from build123d import *

# Parameters (mm, degrees)
SKETCH1_W                        = 35
SKETCH1_H                        = 38
BASE_FLANGE1_DEPTH               = 2
TAP_DRILL_FOR_M3X0_5_TAP1_D      = 2.5
FILLET1_R                        = 3
TAP_DRILL_FOR_M10X1_5_TAP1_D     = 8.5
TAP_DRILL_FOR_M10X1_5_TAP1_DEPTH = 5
TAP_DRILL_FOR_M10X1_5_TAP1_TIP   = 2.553657631


# Sheet-metal steps are written as plain solids
with BuildPart() as part:
    # Sketch1 → Base-Flange1 (new body)
    with BuildSketch(Plane(origin=(0, 0, 0), x_dir=(1, 0, 0), z_dir=(0, 1, 0))):
        Rectangle(SKETCH1_W, SKETCH1_H)
    extrude(amount=-BASE_FLANGE1_DEPTH)

    # Tap Drill for M3x0.5 Tap1 (through all)
    with Locations(Plane(origin=(0, 0, 0), x_dir=(1, 0, 0), z_dir=(0, 1, 0))):
        with Locations((-9.5, -13), (-9.5, 13)):
            Hole(TAP_DRILL_FOR_M3X0_5_TAP1_D / 2)

    # Fillet1
    fillet1_edges = [part.edges().sort_by_distance(p)[0] for p in [
        (-17.5, -1, -19),
        (17.5, -1, -19),
        (17.5, -1, 19),
        (-17.5, -1, 19),
    ]]
    fillet(fillet1_edges, radius=FILLET1_R)

    # Tap Drill for M10x1.5 Tap1
    with Locations(Plane(origin=(0, 0, 0), x_dir=(1, 0, 0), z_dir=(0, 1, 0))):
        with Locations((9.5, 0)):
            Hole(TAP_DRILL_FOR_M10X1_5_TAP1_D / 2, depth=TAP_DRILL_FOR_M10X1_5_TAP1_DEPTH)
            with Locations((0, 0, -(TAP_DRILL_FOR_M10X1_5_TAP1_DEPTH + TAP_DRILL_FOR_M10X1_5_TAP1_TIP / 2))):  # 118° drill point
                Cone(0, TAP_DRILL_FOR_M10X1_5_TAP1_D / 2, TAP_DRILL_FOR_M10X1_5_TAP1_TIP, mode=Mode.SUBTRACT)


solid = part.part
Verification items for the finished model (mm, model axes). Coordinates: 2 decimals unless noted, no trailing zeros. Write each loop counter-clockwise with the first axis right and the second up, starting at its lowest first coordinate (ties: lowest second). Pieces come first, ordered by that corner, then holes. Notation, with made-up numbers: M -39,76.25 L -10,76.25 A12 ccw -10,97.25 Z; hole C -34.5,-1.5 d8. An arc over 180 degrees is marked long. Use a Markdown table: item, result.
Q1. Sectioned sample at C-C, the plane y = -1.3. Record the boundary of the cut face in (x, z), plus the area to 3 significant figures.
Reply:
| item | result |
|---|---|
| outline | M -17.5,-16 A3 ccw -14.5,-19 L 14.5,-19 A3 ccw 17.5,-16 L 17.5,16 A3 ccw 14.5,19 L -14.5,19 A3 ccw -17.5,16 Z; hole C -9.5,-13 d2.5; hole C -9.5,13 d2.5; hole C 9.5,0 d8.5 |
| area | 1,260 mm² |
Q2. Sectioned sample at D-D, the plane x = -9.5. Record the boundary of the cut face in (y, z).
Reply:
| item | result |
|---|---|
| outline | M -2,-19 L 0,-19 L 0,-14.25 L -2,-14.25 Z; M -2,-11.75 L 0,-11.75 L 0,11.75 L -2,11.75 Z; M -2,14.25 L 0,14.25 L 0,19 L -2,19 Z |
Q3. Sectioned sample at A-A, the plane z = 0. Record the boundary of the cut face in (x, y).
Reply:
| item | result |
|---|---|
| outline | M -17.5,-2 L 5.25,-2 L 5.25,0 L -17.5,0 Z; M 13.75,-2 L 17.5,-2 L 17.5,0 L 13.75,0 Z |
Q4. Draft check along X on faces 1 (the face through (-8.579, -1.014, -13.845)), 2 (the face through (7.215, -1.014, -3.584)), 3 (the face through (-16.64, -1.01, -18.1)), 4 (the face through (17.5, -1, 0)). Enter one of: +X half, -X half, draft (parallel to the pull), parting line (faces both ways), or undercut.
Reply:
| item | result |
|---|---|
| face 1 | undercut |
| face 2 | undercut |
| face 3 | -X half |
| face 4 | +X half |
Q5. Thickness scan on line 1 (Z direction, x = -9.5, y = -0.8); line 2 (X direction, y = -1.05, z = -13); line 3 (Z direction, x = 9.5, y = -0.55). Record the ranges inside material, lowest first.
Reply:
| item | result |
|---|---|
| line 1 | z = -19 to -14.25, -11.75 to 11.75, 14.25 to 19 |
| line 2 | x = -17.5 to -10.75, -8.25 to 17.5 |
| line 3 | z = -19 to -4.25, 4.25 to 19 |
Q6. Sectioned sample at B-B, the plane x = 9.5. Record the boundary of the cut face in (y, z), plus the area to 3 significant figures.
Reply:
| item | result |
|---|---|
| outline | M -2,-19 L 0,-19 L 0,-4.25 L -2,-4.25 Z; M -2,4.25 L 0,4.25 L 0,19 L -2,19 Z |
| area | 59.0 mm² |
Q7. Go/stop test with a flat-tipped pin: P1, Ø1.5, axis at x = -9.5, z = -13, coming from the +Y side. Record where the tip stops, or that it passes through.
Reply:
| item | result |
|---|---|
| P1 | passes through |
